Check sheet for the drawn part. Datum: minimum x, y, z corner. Units: mm. Round coordinates to 2 decimals unless told otherwise and drop trailing zeros. Order: outer loops, then holes, each group sorted by start corner. A loop starts at its lowest first (then second) coordinate and runs counter-clockwise, first axis right, second up.
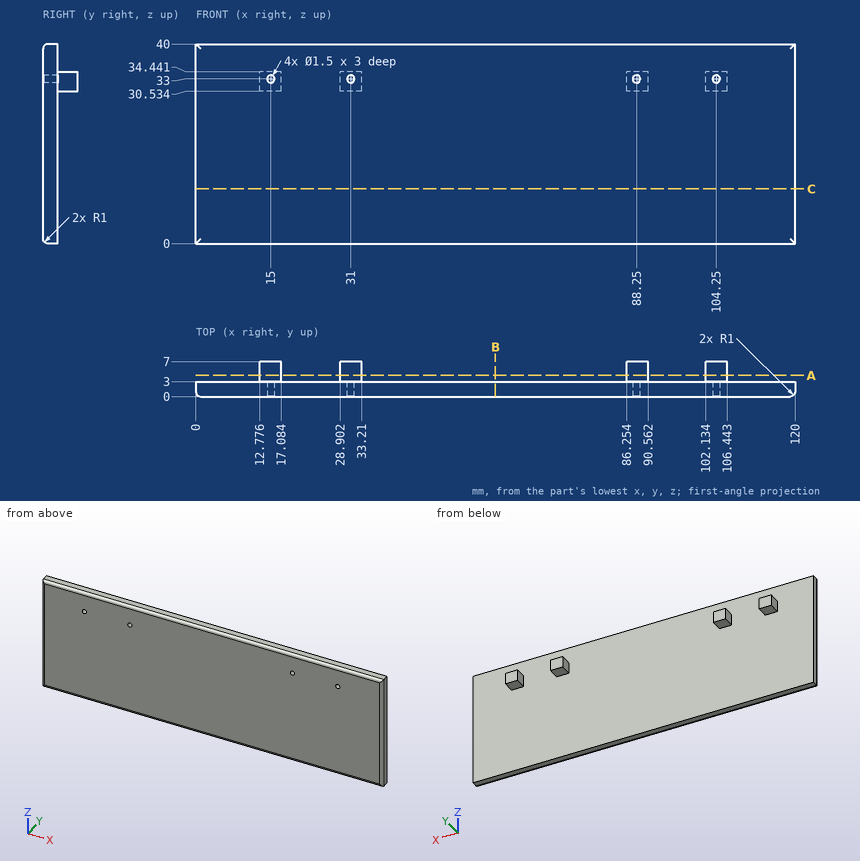
(1) Material ranges on line 1 (X direction, y = 2, z = 33); line 2 (Z direction, x = 31, y = 2.1); line 3 (Y direction, x = 113.5, z = 11.5), recorded low to high.
Returned:
line 1: x = 0 to 14.25, 15.75 to 30.25, 31.75 to 87.5, 89 to 103.5, 105 to 120
line 2: z = 0 to 32.25, 33.75 to 40
line 3: y = 0 to 3
(2) Sectioned sample at C-C, the plane z = 11. Record the cut outline in (x, y).
Returned:
outline: (0, 1) arc R1 ccw to (1, 0) - (119, 0) arc R1 ccw to (120, 1) - (120, 3) - (0, 3) - close
(3) Depth check by flat-ended pin: P1, Ø1.2, axis at x = 88, y = 6, coming from the +Z side; P2, Ø2, axis at y = 5.5, z = 32, coming from the -X side; P3, Ø1.2, axis at y = 4, z = 31.5, coming from the +X side. Enter the tip coordinate at first touch or a pass-through.
Returned:
P1: stops at z = 34.44
P2: stops at x = 12.78
P3: stops at x = 106.44
(4) Sectioned sample at A-A, the plane y = 4.25. Record the cut outline in (x, z) (1 decimal).
Returned:
outline: (12.8, 30.5) - (17.1, 30.5) - (17.1, 34.4) - (12.8, 34.4) - close; (28.9, 30.5) - (33.2, 30.5) - (33.2, 34.4) - (28.9, 34.4) - close; (86.3, 30.5) - (90.6, 30.5) - (90.6, 34.4) - (86.3, 34.4) - close; (102.1, 30.5) - (106.4, 30.5) - (106.4, 34.4) - (102.1, 34.4) - close
(5) Sectioned sample at B-B, the plane x = 60. Record the cut outline in (y, z).
Returned:
outline: (0, 1) arc R1 ccw to (1, 0) - (3, 0) - (3, 40) - (1, 40) arc R1 ccw to (0, 39) - close
